Autodesk Inventor part; units mm, degrees
ref_plane "YZ Plane" through (0, 0, 0) normal (1, 0, 0) x (0, 1, 0)
ref_plane "XZ Plane" through (0, 0, 0) normal (0, 1, 0) x (-1, 0, 0)
ref_plane "XY Plane" through (0, 0, 0) normal (0, 0, 1) x (1, 0, 0)
sketch "Sketch1" plane through (0, 0, 0) normal (0, 0, 1) x (1, 0, 0)
  line L0 (0, 0) -> (95, 0)
  line L1 (95, 0) -> (95, 20)
  line L2 (95, 20) -> (0, 20)
  line L3 (0, 20) -> (0, 0)
  dimension "d0" = 95
  dimension "d1" = 20
extrude "Extrusion1" add sketch "Sketch1" along normal blind 400
sketch "Sketch4" plane through (0, 20, 0) normal (0, 1, 0) x (1, 0, 0)
  line L0 (95, 0) -> (0, 0)
  line L1 (0, 0) -> (0, -400)
  line L2 (95, -400) -> (0, -400)
  line L3 (95, 0) -> (95, -400)
  line L4 (95, -376.825) -> (95, -383.175)
  line L5 (0, -383.175) -> (0, -376.825)
  line L6 (95, 0) -> (72.5, 0)
  line L7 (72.5, 0) -> (72.5, -310)
  line L8 (72.5, -310) -> (95, -310)
  line L9 (95, -310) -> (95, 0)
  line L10 (0, 0) -> (22.5, 0)
  line L11 (22.5, 0) -> (22.5, -310)
  line L12 (22.5, -310) -> (0, -310)
  line L13 (0, -310) -> (0, 0)
  dimension "d30" = 90
  dimension "d31" = 50
  dimension "d32" = 22.5
extrude "Extrusion4" cut sketch "Sketch4" against normal up to next contours L3 L8 L7 L0 | L11 L12 L1 L0
sketch "Sketch5" plane through (0, 20, 400) normal (0, 1, 0) x (1, 0, 0)
  circle A0 centre (62.5, 360) radius 2.5
  circle A1 centre (32.5, 360) radius 2.5
  circle A2 centre (62.5, 390) radius 2.5
  circle A3 centre (32.5, 390) radius 2.5
  line L0 (22.5, 400) -> (22.5, 90)
  line L1 (22.5, 90) -> (0, 90)
  line L2 (0, 90) -> (0, 0)
  line L3 (95, 0) -> (0, 0)
  line L4 (95, 90) -> (95, 0)
  line L5 (95, 90) -> (72.5, 90)
  line L6 (72.5, 90) -> (72.5, 400)
  line L7 (72.5, 400) -> (22.5, 400)
  point P0 (0, 400)
  dimension "d35" = 5
  dimension "d36" = 5
  dimension "d37" = 5
  dimension "d38" = 5
  dimension "d39" = 30
  dimension "d40" = 30
  dimension "d41" = 10
  dimension "d42" = 10
  dimension "d43" = 30
  dimension "d44" = 30
  dimension "d45" = 10
  dimension "d46" = 10
extrude "Extrusion5" cut sketch "Sketch5" against normal up to next contours A0 | A1 | A2 | A3
sketch "Sketch8" plane through (0, 20, 400) normal (0, 1, 0) x (1, 0, 0)
  circle A0 centre (30.325, 15) radius 2.425
  circle A1 centre (11.925, 15) radius 2.425
  circle A2 centre (83.075, 15) radius 2.425
  circle A3 centre (64.675, 15) radius 2.425
  line L0 (0, 90) -> (0, 0)
  line L1 (95, 90) -> (95, 0)
  line L2 (95, 0) -> (0, 0)
  point P0 (0, 400)
  dimension "d60" = 4.85
  dimension "d61" = 4.85
  dimension "d62" = 4.85
  dimension "d63" = 4.85
  dimension "d64" = 11.925
  dimension "d65" = 18.4
  dimension "d66" = 11.925
  dimension "d67" = 18.4
  dimension "d68" = 15
  dimension "d69" = 15
  dimension "d70" = 15
  dimension "d71" = 15
extrude "Extrusion8" cut sketch "Sketch8" against normal up to next
sketch "Sketch9" plane through (0, 20, 400) normal (0, 1, 0) x (1, 0, 0)
  circle A0 centre (43.5, 40) radius 2.15
  circle A1 centre (43.5, 71.8) radius 2.15
  line L0 (95, 0) -> (0, 0)
  line L1 (0, 90) -> (0, 0)
  circle A2 centre (24.5, 40) radius 2.15
  circle A3 centre (24.5, 71.8) radius 2.15
  point P0 (0, 400)
  dimension "d74" = 4.3
  dimension "d75" = 4.3
  dimension "d76" = 31.8
  dimension "d77" = 40
  dimension "d80" = 4.3
  dimension "d81" = 4.3
  dimension "d82" = 19
  dimension "d83" = 19
  dimension "d84" = 31.8
  dimension "d85" = 40
  dimension "d86" = 24.5
  dimension "d87" = 24.5
extrude "Extrusion9" cut sketch "Sketch9" against normal up to next
sketch "Sketch10" plane through (0, 20, 400) normal (0, 1, 0) x (1, 0, 0)
  circle A0 centre (84.5, 55.9) radius 2.5
  circle A1 centre (39.5, 55.9) radius 2.5
  circle A2 centre (24.5, 40) radius 2.15
  circle A3 centre (43.5, 40) radius 2.15
  circle A4 centre (43.5, 71.8) radius 2.15
  circle A5 centre (24.5, 71.8) radius 2.15
  circle A6 centre (83.075, 15) radius 2.425
  circle A7 centre (30.325, 15) radius 2.425
  circle A8 centre (11.925, 15) radius 2.425
  circle A9 centre (64.675, 15) radius 2.425
  circle A10 centre (62.5, 390) radius 2.5
  circle A11 centre (62.5, 360) radius 2.5
  circle A12 centre (32.5, 360) radius 2.5
  circle A13 centre (32.5, 390) radius 2.5
  line L0 (22.5, 400) -> (22.5, 90)
  line L1 (22.5, 90) -> (0, 90)
  line L2 (0, 90) -> (0, 0)
  line L3 (95, 0) -> (0, 0)
  line L4 (95, 90) -> (95, 0)
  line L5 (95, 90) -> (72.5, 90)
  line L6 (72.5, 90) -> (72.5, 400)
  line L7 (72.5, 400) -> (22.5, 400)
  circle A14 centre (62, 55.9) radius 3.175
  point P0 (0, 400)
  dimension "d90" = 45
  dimension "d91" = 5
  dimension "d92" = 5
  dimension "d93" = 15.9
  dimension "d94" = 15.9
  dimension "d95" = 39.5
  dimension "d106" = 6.35
  dimension "d107" = 22.5
  dimension "d108" = 15.9
extrude "Extrusion10" cut sketch "Sketch10" against normal up to next contours A0 | A1 | A14
sketch "Sketch11" plane through (0, 20, 400) normal (0, 1, 0) x (1, 0, 0)
  circle A0 centre (57.5, 300) radius 2.5
  circle A1 centre (37.5, 300) radius 2.5
  line L0 (72.5, 400) -> (22.5, 400)
  line L1 (72.5, 90) -> (72.5, 400)
  point P0 (0, 400)
  dimension "d98" = 5
  dimension "d99" = 5
  dimension "d100" = 20
  dimension "d101" = 100
  dimension "d102" = 100
  dimension "d103" = 15
extrude "Extrusion11" cut sketch "Sketch11" against normal up to next
equation "\"d87\" = d86"
properties part number "Arm-SquareBar-Rev3"
The listing builds one solid part. Answer for the finished solid, in the listing's coordinates (mm). A direction names the side the tool comes from. Round coordinates to 2 decimals unless told otherwise and drop trailing zeros. Write each loop counter-clockwise with the first axis right and the second up, starting at its lowest first coordinate (ties: lowest second). Pieces come first, ordered by that corner, then holes. Notation, with made-up numbers: (34, 43) -> (52, 43) arc R16 cw to (52, 53) -> close; hole circle Ø2 at (19, 51.5). An arc over 180 degrees is marked (long way). Answer as a JSON object with one key per item and string values. Group by question number.
Q1. Each of these flat-tipped pins is pushed along its axis until it touches: pin 1 Ø3.5 at (x, z) = (24.5, 328.2) entering from +Y; pin 2 Ø6 at (x, y) = (86.5, 10.5) entering from -Z; pin 3 Ø4 at (y, z) = (4, 283) entering from +X; pin 4 Ø12 at (y, z) = (16, 287.5) entering from -X. Where does it stop, or does it pass through?
Q2. Determine the mould class of faces 4 (the face through (63.707, 10.14, 341.423)), 5 (the face through (0, 10, 354)), 6 (the face through (84, 10, 310)) for opening direction Z: pulls with the +Z half, pulls with the -Z half, needs draft (parallel to the pull), parting line crosses it, or undercut.
Q3. Section A-A (y = 7.5) is taken. Count the separate pieces of the cut face and the enclosed holes in it, plus the area to 3 significant figures.
Q4. Straight lines are drawn through the part: line 1 along Z through (x, y) = (43.5, 8); line 2 along Z through (x, y) = (57.5, 14.75); line 3 along Z through (x, y) = (37.5, 6). For each, find the intervals that lie inside material, in ascending order.
Q5. Section B-B (z = 222) is taken. Write down the section's boundary in (x, y).
Q6. Which of the six approach directions +Z, -Z, +X, -X, +Y, -Y give full straight-line access (tool end or side, diameter ignored) to faces 1 (the face through (47, 0, 242)), 2 (the face through (22.5, 10, 153)), 3 (the face through (72.5, 10, 153))?
Check values:
{
 "1": {"pin 1": "through", "pin 2": "z = 310", "pin 3": "x = 72.5", "pin 4": "x = 22.5"},
 "2": {"face 4": "undercut", "face 5": "needs draft", "face 6": "pulls with the -Z half"},
 "3": {"separate pieces": "1", "enclosed holes": "17", "area": "23,700 mm^2"},
 "4": {"line 1": "0 to 326.05, 330.35 to 357.85, 362.15 to 400", "line 2": "0 to 97.5, 102.5 to 400", "line 3": "0 to 97.5, 102.5 to 342.6, 345.6 to 400"},
 "5": {"outline": "(22.5, 0) -> (72.5, 0) -> (72.5, 20) -> (22.5, 20) -> close"},
 "6": {"face 1": "+Z, -Z, +X, -X, -Y", "face 2": "-Z, -X, +Y, -Y", "face 3": "-Z, +X, +Y, -Y"}
}
